Autodesk Inventor part; units mm, degrees
ref_plane "YZ Plane" through (0, 0, 0) normal (1, 0, 0) x (0, 1, 0)
ref_plane "XZ Plane" through (0, 0, 0) normal (0, 1, 0) x (-1, 0, 0)
ref_plane "XY Plane" through (0, 0, 0) normal (0, 0, 1) x (1, 0, 0)
sketch "Sketch1" plane through (0, 0, 0) normal (1, 0, 0) x (0, 1, 0)
  line L0 (-76.2, 76.2) -> (76.2, 76.2)
  line L1 (76.2, 76.2) -> (76.2, -76.2)
  line L2 (76.2, -76.2) -> (-76.2, -76.2)
  line L3 (-76.2, -76.2) -> (-76.2, 76.2)
  circle A0 centre (62.8611, 62.86) radius 2.032
  circle A1 centre (-62.8625, -62.8636) radius 2.032
  circle A2 centre (-0.0007, -88.9018) radius 2.032
  circle A3 centre (-62.8625, 62.86) radius 2.032
  circle A4 centre (88.8993, -0.0018) radius 2.032
  circle A5 centre (-88.9007, -0.0018) radius 2.032
  circle A6 centre (62.8611, -62.8636) radius 2.032
  circle A7 centre (-0.0007, 88.8982) radius 2.032
  circle A8 centre (-0.0007, -0.0018) radius 6.35
  dimension "d0" = 152.4
  dimension "d1" = 152.4
  dimension "d5" = 12.7
extrude "Extrusion2" add sketch "Sketch1" along normal blind 3.175 contours L0 L1 L2 L3 | A8
fillet "Fillet2" radius 3.175 4 edges at (1.5875, 76.2, 76.2) (1.5875, 76.2, -76.2) (1.5875, -76.2, 76.2) (1.5875, -76.2, -76.2)
sketch "Sketch2" plane through (3.175, 0, 0) normal (1, 0, 0) x (0, 0, -1)
  line L0 (-50.8, -50.8) -> (50.8, -50.8)
  line L1 (50.8, -50.8) -> (50.8, 50.8)
  line L2 (50.8, 50.8) -> (-50.8, 50.8)
  line L3 (-50.8, 50.8) -> (-50.8, -50.8)
  line L4 (-50.8, -50.8) -> (50.8, 50.8) construction
  line L5 (50.8, -50.8) -> (-50.8, 50.8) construction
  circle A0 centre (0, 0) radius 12.7
  line L6 (-12.7, 0) -> (-50.8, 38.1)
  line L7 (0, 12.7) -> (-38.1, 50.8)
  line L8 (-38.1, 50.8) -> (0, 12.7)
  line L9 (38.1, 50.8) -> (0, 12.7)
  line L10 (12.7, 0) -> (50.8, 38.1)
  line L11 (12.7, 0) -> (50.8, -38.1)
  line L12 (0, -12.7) -> (38.1, -50.8)
  line L13 (0, -12.7) -> (-38.1, -50.8)
  line L14 (-12.7, 0) -> (-50.8, -38.1)
  dimension "d9" = 101.6
  dimension "d10" = 101.6
  dimension "d11" = 25.4
extrude "Extrusion3" [suppressed]
fillet "Fillet3" [suppressed]
sketch "Sketch4" plane through (0, 0, 0) normal (-1, 0, 0) x (0, 0, 1)
  circle A0 centre (0, 0) radius 12.7
  circle A1 centre (50.8, 0) radius 12.7
  circle A2 centre (-50.8, 0) radius 12.7
  dimension "d18" = 25.4
  dimension "d21" = 25.4
  dimension "d22" = 25.4
  dimension "d23" = 50.8
  dimension "d24" = 50.8
extrude "Extrusion6" cut sketch "Sketch4" against normal blind 25.4
properties part number "Bottom Plate"
The model under review builds one solid part; all positions refer to its coordinate system, in mm. Give positions to 0.01 mm unless a question says otherwise; leave off trailing zeros. Order: outer loops, then holes, each group sorted by start corner. A loop starts at its lowest first (then second) coordinate and runs counter-clockwise, first axis right, second up. Notation, with made-up numbers: (20, 73) - (76, 73) arc R25 cw to (76, 95) - close; hole circle Ø11 at (82.5, 85). An arc over 180 degrees is marked (long way). Use CSV: the item, a comma, the result in double quotes. Start each with the question number.
Q1. Clearance check with a flat-ended pin moving along its axis: pin 1 Ø6 at (y, z) = (-9, 12) entering from -X. State where the tip first meets the part, or that it passes through.
Q2. The part is to be moulded in two halves that separate along Z. For faces 1 (the flat face through (3.175, 16, 1)), 2 (the cylindrical face through (1.57, 64.8, 62.25)), say which applies: +Z half, -Z half, draft (parallel to the pull), parting line (faces both ways), or undercut.
Q3. We need section D-D, the plane z = -9.5. Write out the cut boundary in (x, y) (3 decimals).
Q4. We need section C-C, the plane x = 0.6. State how many separate pieces and enclosed holes the cut face has, and give its area (3 significant figures).
Q5. To check wall thickness, follow line 1 along Y through (x, z) = (2.45, 0); line 2 along Y through (x, z) = (0.2, 41); line 3 along Z through (x, y) = (0.8, 7). State the ranges of each line that lie inside material, in increasing order. Write a range as [from, to].
Q6. We need section A-A, the plane y = 0. Write out the cut boundary in (x, z) (3 decimals).
Q7. We need section B-B, the plane z = 50.8. Write out the cut boundary in (x, y) (3 decimals), and give its area (3 significant figures).
Outcome:
1,pin 1,"stops at x = 0"
2,face 1,"draft"
2,face 2,"undercut"
3,outline,"(0, -76.2) - (3.175, -76.2) - (3.175, -8.429) - (0, -8.429) - close; (0, 8.429) - (3.175, 8.429) - (3.175, 76.2) - (0, 76.2) - close"
4,separate pieces,"1"
4,enclosed holes,"7"
4,area,"21,600 mm^2"
5,line 1,"y = [-76.2, -12.7], [12.7, 76.2]"
5,line 2,"y = [-76.2, -8.08], [8.08, 76.2]"
5,line 3,"z = [-76.2, -61.4], [-40.2, -10.6], [10.6, 40.2], [61.4, 76.2]"
6,outline,"(0, -76.2) - (3.175, -76.2) - (3.175, -63.5) - (0, -63.5) - close; (0, -38.1) - (3.175, -38.1) - (3.175, -12.7) - (0, -12.7) - close; (0, 12.7) - (3.175, 12.7) - (3.175, 38.1) - (0, 38.1) - close; (0, 63.5) - (3.175, 63.5) - (3.175, 76.2) - (0, 76.2) - close"
7,outline,"(0, -76.2) - (3.175, -76.2) - (3.175, -12.7) - (0, -12.7) - close; (0, 12.7) - (3.175, 12.7) - (3.175, 76.2) - (0, 76.2) - close"
7,area,"403 mm^2"
